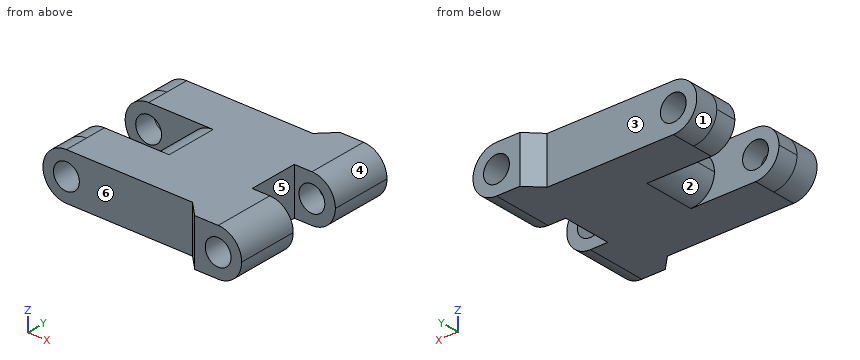
Autodesk Inventor part; units mm, degrees
ref_plane "Work Plane1" through (-9, 0, 0) normal (1, 0, 0) x (0, 0, -1)
ref_plane "Work Plane2" through (-3.5, 4, 0) normal (0, 1, 0) x (1, 0, 0)
ref_plane "Work Plane3" through (0, 4, 0) normal (0, 1, 0) x (1, 0, 0)
sketch "Sketch1" plane through (0, 0, 0) normal (0, 1, 0) x (-1, 0, 0)
  line L0 (0, 0) -> (18, 0)
  line L1 (18, 0) -> (18, -4)
  line L2 (18, -4) -> (0, -4)
  line L3 (0, -4) -> (0, 0)
  line L4 (18, -2) -> (16, -2)
  line L5 (9, -4) -> (9, -3)
  circle A0 centre (16, -2) radius 1.1
  circle A1 centre (2, -2) radius 1.1
  dimension "d0" = 18
  dimension "d1" = 4
  dimension "d2" = 2
  dimension "d3" = 2.2
sketch "Sketch1 outline for Extrusion1" plane through (0, 0, 0) normal (0, 1, 0) x (-1, 0, 0)
  line L0 (18, -4) -> (18, 0)
  line L1 (0, -4) -> (18, -4)
  line L2 (0, 0) -> (0, -4)
  line L3 (18, 0) -> (0, 0)
extrude "Extrusion1" add sketch "Sketch1 outline for Extrusion1" along normal blind 8
sketch "Sketch2" plane through (0, 0, -4) normal (0, 0, -1) x (-1, 0, 0)
  line L0 (18, 0) -> (18, 8)
  line L1 (18, 8) -> (18, 6.1)
  line L2 (18, 0) -> (0, 0)
  line L3 (18, 0) -> (18, 1.9)
  line L4 (18, 6.1) -> (14.5, 6.1)
  line L5 (14.5, 6.1) -> (14.5, 1.9)
  line L6 (14.5, 1.9) -> (18, 1.9)
  line L7 (18, 1.9) -> (18, 6.1)
  dimension "d6" = 1.9
  dimension "d7" = 1.9
  dimension "d8" = 3.5
sketch "Sketch2 outline for Extrusion2" plane through (0, 0, -4) normal (0, 0, -1) x (-1, 0, 0)
  line L0 (14.5, 6.1) -> (14.5, 1.9)
  line L1 (18, 6.1) -> (14.5, 6.1)
  line L2 (18, 1.9) -> (18, 6.1)
  line L3 (14.5, 1.9) -> (18, 1.9)
extrude "Extrusion2" cut sketch "Sketch2 outline for Extrusion2" against normal blind 8
ref_plane "Work Plane1" through (-9, 0, 0) normal (1, 0, 0) x (0, 0, -1)
mirror "Mirror1" about plane through (-9, 0, 0) normal (1, 0, 0) of "Extrusion2"
sketch "Sketch1 outline for Extrusion3" plane through (0, 0, 0) normal (0, 1, 0) x (-1, 0, 0)
  circle A0 centre (2, -2) radius 1.1
  circle A1 centre (16, -2) radius 1.1
extrude "Extrusion3" cut sketch "Sketch1 outline for Extrusion3" along normal blind 8
sketch "Sketch4" plane through (0, 8, 0) normal (0, 1, 0) x (1, 0, 0)
  line L0 (-18, 0) -> (0, 0)
  line L1 (0, 0) -> (-4, 0)
  line L2 (-4, 0) -> (-4, 4)
  line L3 (-4, 4) -> (0, 4)
  line L4 (0, 4) -> (0, 0)
  circle A0 centre (-2, 2) radius 1.1
  circle A1 centre (-2, 2) radius 1.1
  dimension "d14" = 4
  dimension "d15" = 4
  dimension "d16" = 2.2
sketch "Sketch4 outline for Extrusion4" plane through (0, 8, 0) normal (0, 1, 0) x (1, 0, 0)
  line L0 (0, 0) -> (0, 4)
  line L1 (-4, 0) -> (0, 0)
  line L2 (0, 4) -> (-4, 4)
  line L3 (-4, 4) -> (-4, 0)
  circle A0 centre (-2, 2) radius 1.1
extrude "Extrusion4" add sketch "Sketch4 outline for Extrusion4" along normal blind 3.25
ref_plane "Work Plane2" through (-3.5, 4, 0) normal (0, 1, 0) x (1, 0, 0)
mirror "Mirror2" about plane through (-3.5, 4, 0) normal (0, 1, 0) of "Extrusion4"
fillet "Fillet2" radius 2 8 edges at (0, 8.675, -4) (0, -0.675, -4) (0, -0.675, 0) (0, 8.675, 0) (-18, 7.05, -4) (-18, 0.95, -4) (-18, 7.05, 0) (-18, 0.95, 0)
chamfer "Chamfer1" distance 3.25 angle 45 2 edges at (-4, 8, -2) (-4, 0, -2)
sketch "Sketch5" plane through (-14.5, 1.9, 0) normal (0, 0, 1) x (1, 0, 0)
  line L0 (0, 4.2) -> (0, 0)
  line L1 (0, 4.2) -> (2, 4.2)
  line L2 (2, 4.2) -> (2, 0)
  line L3 (2, 0) -> (0, 0)
  line L4 (0, 0) -> (0, 4.2)
  point P0 (14.5, -1.9)
  point P1 (0, 0)
  dimension "d23" = 2
sketch "Sketch5 outline for Extrusion5" plane through (-14.5, 1.9, 0) normal (0, 0, 1) x (1, 0, 0)
  line L0 (0, 0) -> (2, 0)
  line L1 (0, 4.2) -> (0, 0)
  line L2 (2, 4.2) -> (0, 4.2)
  line L3 (2, 0) -> (2, 4.2)
extrude "Extrusion5" cut sketch "Sketch5 outline for Extrusion5" against normal blind 20
sketch "Sketch6" plane through (0, 8, 0) normal (0, 1, 0) x (1, 0, 0)
  line L0 (-7.25, 4) -> (-4, 4)
  line L1 (-16, 0) -> (-12.5, 0)
  line L2 (-7.25, 4) -> (-16, 4)
  line L3 (-16, 4) -> (-16, 0)
  line L4 (-16, 0) -> (-7.25, 0)
  line L5 (-7.25, 0) -> (-7.25, 4)
  circle A0 centre (-16, 2) radius 2
  circle A1 centre (-16, 2) radius 1.1
  point P0 (0, 0)
sketch "Sketch6 outline for Extrusion6" plane through (0, 8, 0) normal (0, 1, 0) x (1, 0, 0)
  arc A0 (-16, 4) -> (-16, 0) centre (-16, 2) ccw
  line L0 (-7.25, 4) -> (-16, 4)
  line L1 (-16, 0) -> (-12.5, 0)
  line L2 (-7.25, 0) -> (-7.25, 4)
  line L3 (-12.5, 0) -> (-7.25, 0)
  circle A1 centre (-16, 2) radius 1.1
extrude "Extrusion6" add sketch "Sketch6 outline for Extrusion6" along normal blind 2
sketch "Sketch7" plane through (-3.5, 1.9, -4) normal (0, 0, -1) x (-1, 0, 0)
  line L0 (3.75, 6.1) -> (3.75, 8.1)
  line L1 (3.75, 8.1) -> (1.311143, 8.1)
  line L2 (1.311143, 8.1) -> (1.311143, 4.926567)
  line L3 (1.311143, 4.926567) -> (3.75, 4.926567)
  line L4 (3.75, 4.926567) -> (3.75, 8.1)
  point P0 (-3.5, -1.9)
sketch "Sketch7 outline for Extrusion7" plane through (-3.5, 1.9, -4) normal (0, 0, -1) x (-1, 0, 0)
  line L0 (1.311143, 4.926567) -> (3.75, 4.926567)
  line L1 (1.311143, 8.1) -> (1.311143, 4.926567)
  line L2 (3.75, 8.1) -> (1.311143, 8.1)
  line L3 (3.75, 6.1) -> (3.75, 8.1)
  line L4 (3.75, 4.926567) -> (3.75, 6.1)
extrude "Extrusion7" add sketch "Sketch7 outline for Extrusion7" against normal blind 4
ref_plane "Work Plane3" through (0, 4, 0) normal (0, 1, 0) x (1, 0, 0)
mirror "Mirror3" about plane through (0, 4, 0) normal (0, 1, 0) of "Extrusion6", "Extrusion7"
sketch "Sketch8" plane through (-3.5, 1.9, -4) normal (0, 0, -1) x (-1, 0, 0)
  line L0 (12.5, 0) -> (14.5, 0)
  line L1 (14.5, 0) -> (14.5, -0.1)
  line L2 (14.5, -3.9) -> (14.5, 0)
  line L3 (14.5, -0.1) -> (8.337258, -0.1)
  line L4 (14.5, 4.2) -> (12.5, 4.2)
  line L5 (14.5, 4.2) -> (14.5, 4.3)
  line L6 (14.5, 4.2) -> (14.5, 8.1)
  line L7 (14.5, 4.3) -> (6.488775, 4.3)
  line L8 (14.5, -0.1) -> (9.5, -0.1)
  line L9 (9.5, -0.1) -> (9.5, 4.3)
  line L10 (9.5, 4.3) -> (14.5, 4.3)
  line L11 (14.5, 4.3) -> (14.5, -0.1)
  point P0 (-3.5, -1.9)
  point P1 (9.5, -0.1)
  dimension "d30" = 0.1
  dimension "d31" = 0.1
sketch "Sketch8 outline for Extrusion8" plane through (-3.5, 1.9, -4) normal (0, 0, -1) x (-1, 0, 0)
  line L0 (14.5, 0) -> (14.5, 4.2)
  line L1 (14.5, -0.1) -> (14.5, 0)
  line L2 (9.5, -0.1) -> (14.5, -0.1)
  line L3 (9.5, 4.3) -> (9.5, -0.1)
  line L4 (14.5, 4.3) -> (9.5, 4.3)
  line L5 (14.5, 4.2) -> (14.5, 4.3)
extrude "Extrusion8" cut sketch "Sketch8 outline for Extrusion8" against normal blind 4
sketch "Sketch9" plane through (-3.5, 1.9, -4) normal (0, 0, -1) x (-1, 0, 0)
  line L0 (12.5, -0.1) -> (9.5, -0.1)
  line L1 (9, 0) -> (9, 4.2)
  line L2 (9.5, -0.1) -> (9, -0.1)
  line L3 (9, -0.1) -> (9, 0)
  line L4 (9, 0) -> (9.5, 0)
  line L5 (9.5, 0) -> (9.5, -0.1)
  line L6 (9, 4.2) -> (9.5, 4.2)
  line L7 (9.5, 4.2) -> (9.5, 4.3)
  line L8 (9, 4.2) -> (9.5, 4.2)
  line L9 (9.5, 4.2) -> (9.5, 4.3)
  line L10 (9.5, 4.3) -> (9, 4.3)
  line L11 (9, 4.3) -> (9, 4.2)
  point P0 (-3.5, -1.9)
sketch "Sketch9 outline for Extrusion9" plane through (-3.5, 1.9, -4) normal (0, 0, -1) x (-1, 0, 0)
  line L0 (9, 4.3) -> (9, 4.2)
  line L1 (9.5, 4.3) -> (9, 4.3)
  line L2 (9.5, 4.2) -> (9.5, 4.3)
  line L3 (9, 4.2) -> (9.5, 4.2)
  line L4 (9, 0) -> (9, -0.1)
  line L5 (9.5, 0) -> (9, 0)
  line L6 (9.5, -0.1) -> (9.5, 0)
  line L7 (9, -0.1) -> (9.5, -0.1)
extrude "Extrusion9" cut sketch "Sketch9 outline for Extrusion9" against normal blind 20
fillet "Fillet3" radius 2 2 edges at (-12.5, 4, -4) (-12.5, 4, 0)
properties part number "short_link_v2"
Source: CAD feature listing. Evaluate the final solid. Frame: model axes, mm. Face numbers are marked on the shaded views. A direction names the side the tool comes from. Coordinates: 2 decimals unless noted, no trailing zeros. Write each loop counter-clockwise with the first axis right and the second up, starting at its lowest first coordinate (ties: lowest second). Pieces come first, ordered by that corner, then holes. Notation, with made-up numbers: M 3.25,55.5 L 47.25,55.5 A20 ccw 47.25,70.5 Z; hole C 28,-25 d10. An arc over 180 degrees is marked long. Use a Markdown table: item, result.
1) First-contact query: pin 1 Ø1.5 at (x, z) = (-10.5, -1.5) entering from -Y; pin 2 Ø1.2 at (x, z) = (-16, -3) entering from +Y. Flat tips, straight axial feed; report the tip coordinate or a pass-through.
Conclusion:
| item | result |
|---|---|
| pin 1 | stops at y = -2 |
| pin 2 | stops at y = 10 |
2) Mould query, pull axis Y, two halves, no side actions, for the marked faces 3, 4, 5 and 6. Classes: pulls with the +Y half, pulls with the -Y half, needs draft (parallel to the pull), parting line crosses it, or undercut.
Conclusion:
| item | result |
|---|---|
| face 3 | pulls with the +Y half |
| face 4 | needs draft |
| face 5 | undercut |
| face 6 | pulls with the -Y half |
3) Section B-B, the plane x = -15.75. Output: boundary loops of the cut face in (y, z).
Conclusion:
| item | result |
|---|---|
| outline | M -2,-4 L 1.8,-4 L 1.8,-3.07 L -2,-3.07 Z; M -2,-0.93 L 1.8,-0.93 L 1.8,0 L -2,0 Z; M 6.2,-4 L 10,-4 L 10,-3.07 L 6.2,-3.07 Z; M 6.2,-0.93 L 10,-0.93 L 10,0 L 6.2,0 Z |
4) Reachability of the marked faces 1 and 2 from +Z, -Z, +X, -X, +Y, -Y: full face, straight path, thin tool, end or side. Return the list, or none.
Conclusion:
| item | result |
|---|---|
| face 1 | -X, +Y, -Y |
| face 2 | -Z, -X |
5) Section A-A, the plane y = 1. Give the number of separate pieces and of enclosed holes in the cut face, then the cut area to 3 significant figures.
Conclusion:
| item | result |
|---|---|
| separate pieces | 1 |
| enclosed holes | 2 |
| area | 61.0 mm^2 |
6) Ray query, L1, parallel to X at y = 1.75, z = -1.95; L2, parallel to Y at x = -14, z = -1.3; L3, parallel to Y at x = -1.5, z = -0.45. Return the intervals inside material, ascending.
Conclusion:
| item | result |
|---|---|
| L1 | x = -18 to -17.1, -14.9 to -3.1, -0.9 to 0 |
| L2 | y = -2 to 1.8, 6.2 to 10 |
| L3 | y = -3.25 to 1.9, 6.1 to 11.25 |
